from build123d import *

# Parameters (mm, degrees)
F0_W     = 20
F0_H     = 32
F0_R     = 3.75
F1_DEPTH = 2
F2_DEPTH = 10
F3_DEPTH = 4


with BuildPart() as f1:
    # F0 (on Top) → F1 (new body)
    with BuildSketch(Plane.XY):
        Polygon((12, 4), (12, 18), (4, 18), (-4, 18), (-12, 18), (-12, 4), (-12, -4), (-12, -18), (-4, -18), (4, -18), (12, -18), (12, -4), align=None)
        Rectangle(F0_W, F0_H, mode=Mode.SUBTRACT)
        Rectangle(F0_W, F0_H)
        with BuildLine():
            Line((-12, 18), (-4, 18))
            Line((-4, 18), (-26, 34.1306779105))
            ThreePointArc((-26, 34.1306779105), (-24.7055453539, 32.2430448056), (-24.25, 30))
            ThreePointArc((-24.25, 30), (-27.1072816845, 25.0306257188), (-32.8394541729, 25))
            Line((-32.8394541729, 25), (-12, 4))
            Line((-12, 4), (-12, 18))
        make_face()
        with BuildLine():
            Line((4, 18), (12, 18))
            Line((12, 18), (12, 4))
            Line((12, 4), (32.8394541729, 25))
            ThreePointArc((32.8394541729, 25), (25.397931288, 26.552760007), (26, 34.1306779105))
            Line((26, 34.1306779105), (4, 18))
        make_face()
        with BuildLine():
            Line((32.8394541729, -25), (12, -4))
            Line((12, -4), (12, -18))
            Line((12, -18), (4, -18))
            Line((4, -18), (26, -34.1306779105))
            ThreePointArc((26, -34.1306779105), (25.397931288, -26.552760007), (32.8394541729, -25))
        make_face()
        with BuildLine():
            Line((-12, -18), (-12, -4))
            Line((-12, -4), (-32.8394541729, -25))
            ThreePointArc((-32.8394541729, -25), (-27.1072816845, -25.0306257188), (-24.25, -30))
            ThreePointArc((-24.25, -30), (-24.7055453539, -32.2430448056), (-26, -34.1306779105))
            Line((-26, -34.1306779105), (-4, -18))
            Line((-4, -18), (-12, -18))
        make_face()
        with BuildLine():
            ThreePointArc((-24.25, 30), (-24.7055453539, 32.2430448056), (-26, 34.1306779105))
            ThreePointArc((-26, 34.1306779105), (-34.602068712, 33.447239993), (-32.8394541729, 25))
            ThreePointArc((-32.8394541729, 25), (-27.1072816845, 25.0306257188), (-24.25, 30))
        make_face()
        with Locations((-30, 30)):
            Circle(F0_R, mode=Mode.SUBTRACT)
        with BuildLine():
            ThreePointArc((35.75, 30), (32.2430448056, 35.2944546461), (26, 34.1306779105))
            ThreePointArc((26, 34.1306779105), (25.397931288, 26.552760007), (32.8394541729, 25))
            ThreePointArc((32.8394541729, 25), (34.9693742812, 27.1072816845), (35.75, 30))
        make_face()
        with Locations((30, 30)):
            Circle(F0_R, mode=Mode.SUBTRACT)
        with BuildLine():
            ThreePointArc((-24.25, -30), (-27.1072816845, -25.0306257188), (-32.8394541729, -25))
            ThreePointArc((-32.8394541729, -25), (-34.602068712, -33.447239993), (-26, -34.1306779105))
            ThreePointArc((-26, -34.1306779105), (-24.7055453539, -32.2430448056), (-24.25, -30))
        make_face()
        with Locations((-30, -30)):
            Circle(F0_R, mode=Mode.SUBTRACT)
    extrude(amount=F1_DEPTH)

    # F0 (on Top) → F2 (join)
    with BuildSketch(Plane.XY):
        with BuildLine():
            ThreePointArc((-24.25, 30), (-24.7055453539, 32.2430448056), (-26, 34.1306779105))
            ThreePointArc((-26, 34.1306779105), (-34.602068712, 33.447239993), (-32.8394541729, 25))
            ThreePointArc((-32.8394541729, 25), (-27.1072816845, 25.0306257188), (-24.25, 30))
        make_face()
        with Locations((-30, 30)):
            Circle(F0_R, mode=Mode.SUBTRACT)
        with BuildLine():
            ThreePointArc((35.75, 30), (32.2430448056, 35.2944546461), (26, 34.1306779105))
            ThreePointArc((26, 34.1306779105), (25.397931288, 26.552760007), (32.8394541729, 25))
            ThreePointArc((32.8394541729, 25), (34.9693742812, 27.1072816845), (35.75, 30))
        make_face()
        with Locations((30, 30)):
            Circle(F0_R, mode=Mode.SUBTRACT)
        with BuildLine():
            ThreePointArc((35.75, -30), (34.9693742812, -27.1072816845), (32.8394541729, -25))
            ThreePointArc((32.8394541729, -25), (25.397931288, -26.552760007), (26, -34.1306779105))
            ThreePointArc((26, -34.1306779105), (32.2430448056, -35.2944546461), (35.75, -30))
        make_face()
        with Locations((30, -30)):
            Circle(F0_R, mode=Mode.SUBTRACT)
        with BuildLine():
            ThreePointArc((-24.25, -30), (-27.1072816845, -25.0306257188), (-32.8394541729, -25))
            ThreePointArc((-32.8394541729, -25), (-34.602068712, -33.447239993), (-26, -34.1306779105))
            ThreePointArc((-26, -34.1306779105), (-24.7055453539, -32.2430448056), (-24.25, -30))
        make_face()
        with Locations((-30, -30)):
            Circle(F0_R, mode=Mode.SUBTRACT)
    extrude(amount=F2_DEPTH)

    # F0 (on Top) → F3 (join)
    with BuildSketch(Plane.XY):
        Polygon((12, 4), (12, 18), (4, 18), (-4, 18), (-12, 18), (-12, 4), (-12, -4), (-12, -18), (-4, -18), (4, -18), (12, -18), (12, -4), align=None)
        Rectangle(F0_W, F0_H, mode=Mode.SUBTRACT)
    extrude(amount=F3_DEPTH)


solid = f1.part
Work out the finished part from the listing and answer in its coordinate system (mm). A direction names the side the tool comes from. Round coordinates to 2 decimals unless told otherwise and drop trailing zeros. Write each loop counter-clockwise with the first axis right and the second up, starting at its lowest first coordinate (ties: lowest second). Pieces come first, ordered by that corner, then holes. Notation, with made-up numbers: (38, -1.5) - (86, -1.5) arc R7 cw to (86, 9.5) - close; hole circle Ø4 at (36.25, 48). An arc over 180 degrees is marked (long way). Answer in a Markdown table with one row per item. Add a question column.
1. Find the intervals of material crossed by line 1 along Y through (x, z) = (-30, 7.75); line 2 along Y through (x, z) = (-28.5, 6.5); line 3 along X through (y, z) = (-28, 2.5), in increasing order. Write a range as from..to.
2. For faces 1 (the flat face through (0, -16, 3)), 2 (the flat face through (-22.57, 14.65, 0.99)), 3 (the flat face through (0, 18, 2)), 4 (the flat face through (0, -18, 2)), 5 (the flat face through (15.154, 26.178, 0.986)), determine the directions among +Z, -Z, +X, -X, +Y, -Y from which every point of the face is accessible in a straight line to the end or side of a thin tool.
3. The mould has two halves that part along X. Classify faces 6 (the flat face through (30, 26, 10)), 7 (the flat face through (0, 0, 2)), 8 (the flat face through (22.57, -14.65, 0.99)): +X half, -X half, draft (parallel to the pull), parting line (faces both ways), or undercut.
4. A cutting plane is placed at D-D, the plane y = 13. Determine the outline of the cut face in (x, z), and give its area (3 significant figures).
5. A cutting plane is placed at A-A, the plane z = 7. Determine the outline of the cut face in (x, y).
6. A cutting plane is placed at B-B, the plane y = 30. Determine the outline of the cut face in (x, z), and give its area (3 significant figures).
7. Given pin 1 (8.5 mm diameter, centred on x = -11.5, y = -13, fed in from +Z); pin 2 (1.2 mm diameter, centred on x = -2.5, z = 3, fed in from -Y); pin 3 (1 mm diameter, centred on x = -15.5, y = -25, fed in from +Z), each flat-ended and moving along its own axis, determine where each tip first touches the part or whether it passes through.
8. A cutting plane is placed at C-C, the plane x = -28.5. Determine the outline of the cut face in (y, z), and give its area (3 significant figures).
Worked out:
| question | item | result |
|---|---|---|
| 1 | line 1 | -35.75..-33.75, -26.25..-24.25, 24.25..26.25, 33.75..35.75 |
| 1 | line 2 | -35.55..-33.44, -26.56..-24.45, 24.45..26.56, 33.44..35.55 |
| 1 | line 3 | -35.39..-33.17, -26.83..-24.61, 24.61..26.83, 33.17..35.39 |
| 2 | face 1 | +Z |
| 2 | face 2 | +Z, -Z, -X |
| 2 | face 3 | +Z, +Y |
| 2 | face 4 | +Z, -Y |
| 2 | face 5 | +Z, -Z, +Y |
| 3 | face 6 | draft |
| 3 | face 7 | undercut |
| 3 | face 8 | +X half |
| 4 | outline | (-20.93, 0) - (20.93, 0) - (20.93, 2) - (12, 2) - (12, 4) - (10, 4) - (10, 2) - (-10, 2) - (-10, 4) - (-12, 4) - (-12, 2) - (-20.93, 2) - close |
| 4 | area | 91.7 mm^2 |
| 5 | outline | circle Ø11.5 at (-30, -30); circle Ø11.5 at (-30, 30); circle Ø11.5 at (30, -30); circle Ø11.5 at (30, 30); hole circle Ø7.5 at (-30, -30); hole circle Ø7.5 at (-30, 30); hole circle Ø7.5 at (30, -30); hole circle Ø7.5 at (30, 30) |
| 6 | outline | (-35.75, 0) - (-33.75, 0) - (-33.75, 10) - (-35.75, 10) - close; (-26.25, 0) - (-20.37, 0) - (-20.37, 2) - (-24.25, 2) - (-24.25, 10) - (-26.25, 10) - close; (20.37, 0) - (26.25, 0) - (26.25, 10) - (24.25, 10) - (24.25, 2) - (20.37, 2) - close; (33.75, 0) - (35.75, 0) - (35.75, 10) - (33.75, 10) - close |
| 6 | area | 95.5 mm^2 |
| 7 | pin 1 | z = 4 |
| 7 | pin 2 | y = -18 |
| 7 | pin 3 | z = 2 |
| 8 | outline | (-35.55, 0) - (-33.44, 0) - (-33.44, 10) - (-35.55, 10) - close; (-26.56, 0) - (-20.63, 0) - (-20.63, 2) - (-24.45, 2) - (-24.45, 10) - (-26.56, 10) - close; (20.63, 0) - (26.56, 0) - (26.56, 10) - (24.45, 10) - (24.45, 2) - (20.63, 2) - close; (33.44, 0) - (35.55, 0) - (35.55, 10) - (33.44, 10) - close |
| 8 | area | 99.8 mm^2 |
